Design review of the part built by this model. Coordinates are the model's own, in mm. A direction names the side the tool comes from. Coordinates: 2 decimals unless noted, no trailing zeros. Order: outer loops, then holes, each group sorted by start corner. A loop starts at its lowest first (then second) coordinate and runs counter-clockwise, first axis right, second up. Notation, with made-up numbers: (-19, 41) -> (38, 41) arc R16 cw to (38, 70) -> close; hole circle Ø6 at (-12, 4.25). An arc over 180 degrees is marked (long way). Write item = value, one per line.
```python
from build123d import *

# Parameters (mm, degrees)
CROQUIS2_W              = 60
CROQUIS2_H              = 60
SALIENTE_EXTRUIR1_DEPTH = 50.5
SALIENTE_EXTRUIR3_DEPTH = 50
MATRIZL2_COUNT          = 2
MATRIZL2_PITCH          = 40
CROQUIS5_W              = 10
CROQUIS5_H              = 10
CORTAR_EXTRUIR1_DEPTH   = 89.352985235
MATRIZL3_COUNT          = 2
MATRIZL3_PITCH          = 50
MATRIZC1_COUNT          = 2
MATRIZC1_ANGLE          = 90


with BuildPart() as part:
    # Croquis2 → Saliente-Extruir1 (new body)
    with BuildSketch(Plane(origin=(0, 0, 0), x_dir=(1, 0, 0), z_dir=(0, 1, 0))):
        Rectangle(CROQUIS2_W, CROQUIS2_H)
    extrude(amount=SALIENTE_EXTRUIR1_DEPTH)

    # Croquis4 → Saliente-Extruir3 (add)
    with BuildSketch(Plane.XY.offset(30)):
        Polygon((-26, 57.5), (-14, 57.5), (-16, 50.5), (-24, 50.5), align=None)
    saliente_extruir3 = extrude(amount=-SALIENTE_EXTRUIR3_DEPTH)

    # MatrizL2: Saliente-Extruir3 ×2
    with Locations(*[(i * MATRIZL2_PITCH, 0, 0) for i in range(1, MATRIZL2_COUNT)]):
        add(saliente_extruir3)

    # Croquis5 → Cortar-Extruir1 (cut, through all)
    with BuildSketch(Plane.XY.offset(30)):
        with Locations((-25, 15)):
            Rectangle(CROQUIS5_W, CROQUIS5_H)
    cortar_extruir1 = extrude(amount=-CORTAR_EXTRUIR1_DEPTH, mode=Mode.SUBTRACT)

    # MatrizL3: Cortar-Extruir1 ×2
    with Locations(*[(i * MATRIZL3_PITCH, 0, 0) for i in range(1, MATRIZL3_COUNT)]):
        add(cortar_extruir1, mode=Mode.SUBTRACT)

    # MatrizC1: Cortar-Extruir1 ×2 about axis
    matrizc1_axis = Axis((0, 0, 0), (0, 1, 0))
    for i in range(1, MATRIZC1_COUNT):
        add(cortar_extruir1.rotate(matrizc1_axis, i * MATRIZC1_ANGLE / (MATRIZC1_COUNT - 1)), mode=Mode.SUBTRACT)


solid = part.part
```
(1) Insertion check: pin 1 (6 mm diameter, centred on x = -19.5, z = 5.5, fed in from -Y); pin 2 (2 mm diameter, centred on x = -17.5, y = 54.5, fed in from -Z); pin 3 (18 mm diameter, centred on x = 1.5, z = -10.5, fed in from +Y). Each pin has a flat end and moves straight along its axis. Give the tip position at first contact, or say it passes through.
Report:
pin_1 = 0
pin_2 = -20
pin_3 = 50.5
(2) For faces 1 (the flat face through (-7.1, 10, 20.4)), 2 (the flat face through (-15, 54, 5)), 3 (the flat face through (25, 54, 5)), list the 3-axis set-ups (+Z, -Z, +X, -X, +Y, -Y) from which the entire face can be reached by the end or side of a thin tool; tool diameter is ignored.
Report:
face_1 = +Z
face_2 = +Z, -Z
face_3 = +Z, -Z, +X
(3) We need section C-C (x = -4). Write out the cut boundary in (y, z), and give its area (3 significant figures).
Report:
outline = (0, -30) -> (50.5, -30) -> (50.5, 30) -> (20, 30) -> (20, 20) -> (10, 20) -> (10, 30) -> (0, 30) -> close
area = 2,930 mm²
(4) We need section A-A (z = 24). Write out the cut boundary in (x, y).
Report:
outline = (-30, 0) -> (30, 0) -> (30, 10) -> (-30, 10) -> close; (-30, 20) -> (30, 20) -> (30, 50.5) -> (24, 50.5) -> (26, 57.5) -> (14, 57.5) -> (16, 50.5) -> (-16, 50.5) -> (-14, 57.5) -> (-26, 57.5) -> (-24, 50.5) -> (-30, 50.5) -> close
(5) We need section D-D (z = 8). Write out the cut boundary in (x, y), and give its area (3 significant figures).
Report:
outline = (-30, 0) -> (30, 0) -> (30, 10) -> (20, 10) -> (20, 20) -> (30, 20) -> (30, 50.5) -> (24, 50.5) -> (26, 57.5) -> (14, 57.5) -> (16, 50.5) -> (-16, 50.5) -> (-14, 57.5) -> (-26, 57.5) -> (-24, 50.5) -> (-30, 50.5) -> (-30, 20) -> (-20, 20) -> (-20, 10) -> (-30, 10) -> close
area = 2,970 mm²
(6) We need section B-B (y = 53). Write out the cut boundary in (x, z).
Report:
outline = (-24.71, -20) -> (-15.29, -20) -> (-15.29, 30) -> (-24.71, 30) -> close; (15.29, -20) -> (24.71, -20) -> (24.71, 30) -> (15.29, 30) -> close
(7) For L1, parallel to Y at x = -23.5, z = 11; L2, parallel to Y at x = 4.5, z = 25; L3, parallel to Z at x = 16, y = 11, list the stretches that pass through material, from the lowest coordinate up.
Report:
L1 = 0 to 10, 20 to 57.5
L2 = 0 to 10, 20 to 50.5
L3 = -30 to 20
